The listing builds one solid part. Answer for the finished solid, in the listing's coordinates (mm). A direction names the side the tool comes from. Give positions to 0.01 mm unless a question says otherwise; leave off trailing zeros. Order: outer loops, then holes, each group sorted by start corner. A loop starts at its lowest first (then second) coordinate and runs counter-clockwise, first axis right, second up.
```python
from build123d import *

# Parameters (mm, degrees)
SKETCH_1_W                = 29
SKETCH_1_H                = 29
EXTRUDE_1_DEPTH           = 5
SKETCH_2_W                = 25
SKETCH_2_H                = 25
CUT_EXTRUDE_1_DEPTH       = 3
SKETCH_3_W                = 35
SKETCH_3_H                = 29
EXTRUDE_756_DEPTH         = 25.341167732
HOLE_WIZARD_M4_1_D        = 3.3
HOLE_WIZARD_M4_1_DEPTH    = 10.1
HOLE_WIZARD_M4_1_TIP      = 0.991420021
SKETCH_9_R                = 1
CUT_EXTRUDE_2_DEPTH       = 3
SKETCH_11_W               = 29
SKETCH_11_H               = 5
EXTRUDE_4_DEPTH           = 6
CUT_EXTRUDE_8_DEPTH       = 40.383835
SKETCH_19_W               = 80
SKETCH_19_H               = 25
EXTRUDE_5_DEPTH           = 10
HOLE_WIZARD_1_D           = 6.6
HOLE_WIZARD_1_DEPTH       = 10.1
HOLE_WIZARD_1_CBORE_D     = 11
HOLE_WIZARD_1_CBORE_DEPTH = 6.8
HOLE_WIZARD_1_TIP         = 1.982840043
SKETCH_23_W               = 80
SKETCH_23_H               = 10
EXTRUDE_6_DEPTH           = 2
SKETCH_24_W               = 27
SKETCH_24_H               = 10
CUT_EXTRUDE_9_DEPTH       = 2
MM_1_D                    = 4
MM_1_DEPTH                = 5
MM_1_TIP                  = 1.201721238
CUT_EXTRUDE_10_DEPTH      = 5
SKETCH_28_R               = 1
CUT_EXTRUDE_11_DEPTH      = 2
HOLE_WIZARD_M6_1_D        = 5
HOLE_WIZARD_M6_1_DEPTH    = 10
HOLE_WIZARD_M6_1_TIP      = 1.502151548
CUT_EXTRUDE_12_DEPTH      = 62.837260656
CUT_EXTRUDE_12_DEPTH_BACK = 62.837260656
SKETCH_32_W               = 27
SKETCH_32_H               = 10
CUT_EXTRUDE_13_DEPTH      = 6.5
SKETCH_33_W               = 27
SKETCH_33_H               = 10
CUT_EXTRUDE_14_DEPTH      = 6.5
CUT_EXTRUDE_15_DEPTH      = 5
MM_2_D                    = 4
MM_2_DEPTH                = 5
MM_2_TIP                  = 1.201721238
MM_3_D                    = 4
MM_3_DEPTH                = 5
MM_3_TIP                  = 1.201721238


with BuildPart() as part:
    # 草图1 → 凸台-拉伸1 (new body)
    with BuildSketch(Plane(origin=(0, 0, 0), x_dir=(1, 0, 0), z_dir=(0, 1, 0))):
        Rectangle(SKETCH_1_W, SKETCH_1_H)
    extrude(amount=EXTRUDE_1_DEPTH)

    # 草图2 → 切除-拉伸1 (cut)
    with BuildSketch(Plane.XZ.offset(-5)):
        Rectangle(SKETCH_2_W, SKETCH_2_H)
    extrude(amount=CUT_EXTRUDE_1_DEPTH, mode=Mode.SUBTRACT)

    # 草图3 → Extrude 756 (add)
    with BuildSketch(Plane(origin=(0, 0, 0), x_dir=(-1, 0, 0), z_dir=(0, -1, 0))):
        with Locations((3, 0)):
            Rectangle(SKETCH_3_W, SKETCH_3_H)
    extrude(amount=EXTRUDE_756_DEPTH)

    # M4 螺纹孔1
    with Locations(Plane.ZX.offset(2)):
        with Locations((0, 0)):
            Hole(HOLE_WIZARD_M4_1_D / 2, depth=HOLE_WIZARD_M4_1_DEPTH)
            with Locations((0, 0, -(HOLE_WIZARD_M4_1_DEPTH + HOLE_WIZARD_M4_1_TIP / 2))):  # 118° drill point
                Cone(0, HOLE_WIZARD_M4_1_D / 2, HOLE_WIZARD_M4_1_TIP, mode=Mode.SUBTRACT)

    # 草图9 → 切除-拉伸2 (cut)
    with BuildSketch(Plane(origin=(0, 5, 0), x_dir=(1, 0, 0), z_dir=(0, 1, 0))):
        with Locations((-12.5, 12.5)):
            Circle(SKETCH_9_R)
    extrude(amount=-CUT_EXTRUDE_2_DEPTH, mode=Mode.SUBTRACT)

    # 草图11 → 凸台-拉伸4 (add)
    with BuildSketch(Plane.ZY.offset(14.5)):
        with Locations((0, 2.5)):
            Rectangle(SKETCH_11_W, SKETCH_11_H)
    extrude(amount=EXTRUDE_4_DEPTH)

    # 草图17 → 切除-拉伸8 (cut, through all)
    with BuildSketch(Plane(origin=(0, 5, 0), x_dir=(1, 0, 0), z_dir=(0, 1, 0))):
        Polygon((-20.5, -14.5), (14.5, -14.5), (14.5, 14.5), (12.5, 14.5), (12.5, -12.5), (-20.5, -12.5), align=None)
    extrude(amount=-CUT_EXTRUDE_8_DEPTH, mode=Mode.SUBTRACT)

    # 草图19 → 凸台-拉伸5 (add)
    with BuildSketch(Plane(origin=(0, -25.341167732, 0), x_dir=(-1, 0, 0), z_dir=(0, -1, 0))):
        with Locations((6, 0)):
            Rectangle(SKETCH_19_W, SKETCH_19_H)
    extrude(amount=-EXTRUDE_5_DEPTH)

    # 打孔尺寸(%根据)内六角圆柱头螺钉的类型1
    with Locations(Plane(origin=(-31, -15.341167732, 0), x_dir=(0, 0, 1), z_dir=(0, 1, 0))):
        with Locations((0, 0), (0, 50)):
            CounterBoreHole(HOLE_WIZARD_1_D / 2, HOLE_WIZARD_1_CBORE_D / 2, HOLE_WIZARD_1_CBORE_DEPTH, depth=HOLE_WIZARD_1_DEPTH)
            with Locations((0, 0, -(HOLE_WIZARD_1_DEPTH + HOLE_WIZARD_1_TIP / 2))):  # 118° drill point
                Cone(0, HOLE_WIZARD_1_D / 2, HOLE_WIZARD_1_TIP, mode=Mode.SUBTRACT)

    # 草图23 → 凸台-拉伸6 (add)
    with BuildSketch(Plane(origin=(0, 0, -12.5), x_dir=(-1, 0, 0), z_dir=(0, 0, -1))):
        with Locations((6, -20.341167732)):
            Rectangle(SKETCH_23_W, SKETCH_23_H)
    extrude(amount=EXTRUDE_6_DEPTH)

    # 草图24 → 切除-拉伸9 (cut)
    with BuildSketch(Plane.ZY.offset(46)):
        with Locations((-1, -20.341167732)):
            Rectangle(SKETCH_24_W, SKETCH_24_H)
    extrude(amount=-CUT_EXTRUDE_9_DEPTH, mode=Mode.SUBTRACT)

    # 大小mm 暗销孔1
    with Locations(Plane(origin=(-21, -25.341167732, 0), x_dir=(0, 0, -1), z_dir=(0, -1, 0))):
        with Locations((0, 0)):
            Hole(MM_1_D / 2, depth=MM_1_DEPTH)
            with Locations((0, 0, -(MM_1_DEPTH + MM_1_TIP / 2))):  # 118° drill point
                Cone(0, MM_1_D / 2, MM_1_TIP, mode=Mode.SUBTRACT)

    # 草图27 → 切除-拉伸10 (cut)
    with BuildSketch(Plane.XZ.offset(25.341167732)):
        with BuildLine():
            Line((8.5, 2), (9.5, 2))
            ThreePointArc((9.5, 2), (11.5, 0), (9.5, -2))
            Line((9.5, -2), (8.5, -2))
            ThreePointArc((8.5, -2), (6.5, 0), (8.5, 2))
        make_face()
    extrude(amount=-CUT_EXTRUDE_10_DEPTH, mode=Mode.SUBTRACT)

    # 草图28 → 切除-拉伸11 (cut)
    with BuildSketch(Plane.XY.offset(12.5)):
        with Locations((-6, -5.341167732)):
            Circle(SKETCH_28_R)
    extrude(amount=-CUT_EXTRUDE_11_DEPTH, mode=Mode.SUBTRACT)

    # M6 螺纹孔1
    with Locations(Plane(origin=(-6, -25.341167732, 0), x_dir=(0, 0, -1), z_dir=(0, -1, 0))):
        with Locations((0, 0)):
            Hole(HOLE_WIZARD_M6_1_D / 2, depth=HOLE_WIZARD_M6_1_DEPTH)
            with Locations((0, 0, -(HOLE_WIZARD_M6_1_DEPTH + HOLE_WIZARD_M6_1_TIP / 2))):  # 118° drill point
                Cone(0, HOLE_WIZARD_M6_1_D / 2, HOLE_WIZARD_M6_1_TIP, mode=Mode.SUBTRACT)

    # 草图31 → 切除-拉伸12 (cut, two sides: drawn at the far end of the back side and taken through both)
    with BuildSketch(Plane(origin=(-6.0032, 14.658832268, 10.4718), x_dir=(1, 0, 0), z_dir=(0, 0, 1)).offset(-CUT_EXTRUDE_12_DEPTH_BACK)):
        with BuildLine():
            Line((10.117055245, -31.7), (8.854085532, -31.7))
            Line((8.854085532, -31.7), (6.07517942, -36.564132504))
            Line((6.07517942, -36.564132504), (6.531795149, -36.824999624))
            Line((6.531795149, -36.824999624), (10.275, -36.824999624))
            ThreePointArc((10.275, -36.824999624), (11.025, -37.574999624), (10.275, -38.324999624))
            Line((10.275, -38.324999624), (9.525, -38.324999624))
            Line((9.525, -38.324999624), (9.525, -40))
            Line((9.525, -40), (-9.776101272, -40))
            Line((-9.776101272, -40), (-9.776101272, -38.074384714))
            Line((-9.776101272, -38.074384714), (-10.526101272, -38.074384714))
            ThreePointArc((-10.526101272, -38.074384714), (-11.276101272, -37.324384714), (-10.526101272, -36.574384714))
            Line((-10.526101272, -36.574384714), (-6.501264425, -36.574384714))
            Line((-6.501264425, -36.574384714), (-6.501264425, -36.324384714))
            Line((-6.501264425, -36.324384714), (-9.143201284, -31.7))
            Line((-9.143201284, -31.7), (-10.369175052, -31.7))
            ThreePointArc((-10.369175052, -31.7), (-11.119175052, -30.95), (-10.369175052, -30.2))
            Line((-10.369175052, -30.2), (10.117055245, -30.2))
            ThreePointArc((10.117055245, -30.2), (10.867055245, -30.95), (10.117055245, -31.7))
        make_face()
    extrude(amount=CUT_EXTRUDE_12_DEPTH + CUT_EXTRUDE_12_DEPTH_BACK, mode=Mode.SUBTRACT)

    # 草图32 → 切除-拉伸13 (cut)
    with BuildSketch(Plane.ZY.offset(44)):
        with Locations((-1, -20.341167732)):
            Rectangle(SKETCH_32_W, SKETCH_32_H)
    extrude(amount=-CUT_EXTRUDE_13_DEPTH, mode=Mode.SUBTRACT)

    # 草图33 → 切除-拉伸14 (cut)
    with BuildSketch(Plane(origin=(34, 0, 0), x_dir=(0, 0, -1), z_dir=(1, 0, 0))):
        with Locations((1, -20.341167732)):
            Rectangle(SKETCH_33_W, SKETCH_33_H)
    extrude(amount=-CUT_EXTRUDE_14_DEPTH, mode=Mode.SUBTRACT)

    # 草图35 → 切除-拉伸15 (cut)
    with BuildSketch(Plane.XZ.offset(25.341167732)):
        with BuildLine():
            Line((8.5, -6), (9.5, -6))
            ThreePointArc((9.5, -6), (11.5, -8), (9.5, -10))
            Line((9.5, -10), (8.5, -10))
            ThreePointArc((8.5, -10), (6.5, -8), (8.5, -6))
        make_face()
    extrude(amount=-CUT_EXTRUDE_15_DEPTH, mode=Mode.SUBTRACT)

    # 大小mm 暗销孔2
    with Locations(Plane(origin=(-21, -25.341167732, -8), x_dir=(0, 0, -1), z_dir=(0, -1, 0))):
        with Locations((0, 0)):
            Hole(MM_2_D / 2, depth=MM_2_DEPTH)
            with Locations((0, 0, -(MM_2_DEPTH + MM_2_TIP / 2))):  # 118° drill point
                Cone(0, MM_2_D / 2, MM_2_TIP, mode=Mode.SUBTRACT)

    # 大小mm 暗销孔3
    with Locations(Plane(origin=(-21, -25.341167732, 8), x_dir=(0, 0, -1), z_dir=(0, -1, 0))):
        with Locations((0, 0)):
            Hole(MM_3_D / 2, depth=MM_3_DEPTH)
            with Locations((0, 0, -(MM_3_DEPTH + MM_3_TIP / 2))):  # 118° drill point
                Cone(0, MM_3_D / 2, MM_3_TIP, mode=Mode.SUBTRACT)


solid = part.part
```
1) Find section A-A (y = -18). Write down the section's boundary in (x, z).
Geometry says:
outline: (-37.5, -14.5) - (-14.6, -14.5) - (-14.6, 12.5) - (-37.5, 12.5) - close; (2.3, -14.5) - (27.5, -14.5) - (27.5, 12.5) - (2.3, 12.5) - close; hole circle Ø11 at (-31, 0); hole circle Ø11 at (19, 0)
2) Find section D-D (y = 3.5). Write down the section's boundary in (x, z), then the cut area to 3 significant figures.
Geometry says:
outline: (-20.5, -14.5) - (12.5, -14.5) - (12.5, -12.5) - (-11.5, -12.5) arc R1 cw (long way) to (-12.5, -11.5) - (-12.5, 12.5) - (-20.5, 12.5) - close
area: 264 mm2
3) Given P1, Ø0.9, axis at x = 3, y = 4, coming from the +Z side; P2, Ø1.5, axis at y = -9.5, z = -8.5, coming from the -X side; P3, Ø3, axis at y = -7.5, z = 9.5, coming from the +X side, each flat-ended and moving along its own axis, determine where each tip first touches the part or whether it passes through.
Geometry says:
P1: stops at z = -12.5
P2: stops at x = -20.5
P3: stops at x = 12.5
4) For a pull along Z with two mould halves and no side action, classify faces 6 (the conical face through (-5.57, -14.1, 0.06)), 7 (the flat face through (16, -25.341, 2)) as +Z half, -Z half, draft (parallel to the pull), parting line (faces both ways), or undercut.
Geometry says:
face 6: undercut
face 7: draft
5) Find section C-C (y = -7). Write down the section's boundary in (x, z).
Geometry says:
outline: (-20.5, -14.5) - (12.5, -14.5) - (12.5, 12.5) - (-20.5, 12.5) - close; hole circle Ø3.3 at (0, 0)
6) Straight lines are drawn through the part: probe 1 along Z at (x, y) = (-21, -23.2); probe 2 along X at (y, z) = (-15.5, 0); probe 3 along X at (y, z) = (-4.5, 0). For each, find the intervals that lie inside material, in ascending order.
Geometry says:
probe 1: z = -14.5 to -10, -6 to -2, 2 to 6, 10 to 12.5
probe 2: x = -37.5 to -36.5, -25.5 to -8.5, -3.5 to 13.5, 24.5 to 27.5
probe 3: x = -20.5 to -1.65, 1.65 to 12.5
7) A tool of negligible diameter and unlimited length cuts with its end or side. For faces 1 (the flat face through (-20.5, -5, -1)), 2 (the cylindrical face through (4.864, -16.275, -1.189)), 3 (the cylindrical face through (6.5, -22.9, 0)), 4 (the cylindrical face through (-25.547, -18.694, -0.716)), 5 (the cylindrical face through (15.78, -23.76, 0.72)), from which of +Z, -Z, +X, -X, +Y, -Y can it reach the whole face along a straight path? Write none if from no direction.
Geometry says:
face 1: +Z, -Z, -X, +Y
face 2: +Z, -Z
face 3: -Y
face 4: +Y
face 5: +Y, -Y
8) Find section B-B (x = 19). Write down the section's boundary in (y, z).
Geometry says:
outline: (-25.34, -14.5) - (-15.34, -14.5) - (-15.34, -5.5) - (-22.14, -5.5) - (-22.14, -3.3) - (-25.34, -3.3) - close; (-25.34, 3.3) - (-22.14, 3.3) - (-22.14, 5.5) - (-15.34, 5.5) - (-15.34, 12.5) - (-25.34, 12.5) - close
